CAD build for the part. Positions are in the model's coordinates, mm. A direction names the side the tool comes from. Give positions to 0.01 mm unless a question says otherwise; leave off trailing zeros. Order: outer loops, then holes, each group sorted by start corner. A loop starts at its lowest first (then second) coordinate and runs counter-clockwise, first axis right, second up. Notation, with made-up numbers: M -29,2.25 L 25,2.25 A21 ccw 25,21.25 Z; hole C 63,22.5 d11. An arc over 180 degrees is marked long. Put each result on its own line as item: value. Start each with the question number.
1) Cut at A-A (z = 12). Write the cut outline in (x, y).
2) Two-plate mould, pull along Y, no slides. Class faces 1 (the face through (2, 176, 2)), 2 (the face through (-2, 240, 7)), 3 (the face through (-2, 212, 0)): released by +Y, released by -Y, zero draft, split by the parting line, or undercut.
3) Drill centre lines: line 1 (X direction, y = 175.5, z = 10.25); line 2 (Y direction, x = 36.5, z = 11); line 3 (Z direction, x = 1.5, y = 170). Where is each one in solid material? Low to high. Write a range as [from, to].
4) Pin check, flat tip, straight feed: pin 1 (6.5 mm diameter, centred on x = 36.5, y = -175.5, fed in from -Z). Stop position of the tip, or through.
5) Tool access for faces 4 (the face through (2, -175, 2)), 5 (the face through (-2, 3, 15)): list every direction of +Z, -Z, +X, -X, +Y, -Y with a clear straight run to the whole face (end or side of a thin tool).
```python
from build123d import *

# Parameters (mm, degrees)
SKETCH_1_W          = 307
SKETCH_1_H          = 480
EXTRUDE_1_DEPTH     = 15
SKETCH_2_W          = 307
SKETCH_2_H          = 15
CUT_EXTRUDE_1_DEPTH = 2
CUT_EXTRUDE_2_DEPTH = 286.284507115
HOLE_WIZARD_M6_1_D  = 5


with BuildPart() as part:
    # 草图1 → 凸台-拉伸1 (new body)
    with BuildSketch(Plane.XY):
        Rectangle(SKETCH_1_W, SKETCH_1_H)
    extrude(amount=EXTRUDE_1_DEPTH)

    # 草图2 → 切除-拉伸1 (cut)
    with BuildSketch(Plane(origin=(0, 0, 0), x_dir=(-1, 0, 0), z_dir=(0, 0, -1))):
        with Locations((0, 175.5)):
            Rectangle(SKETCH_2_W, SKETCH_2_H)
        with Locations((0, -175.5)):
            Rectangle(SKETCH_2_W, SKETCH_2_H)
    extrude(amount=-CUT_EXTRUDE_1_DEPTH, mode=Mode.SUBTRACT)

    # 草图3 → 切除-拉伸2 (cut, through all)
    with BuildSketch(Plane(origin=(0, 0, 0), x_dir=(-1, 0, 0), z_dir=(0, 0, -1))):
        with BuildLine():
            ThreePointArc((153.5, -76.852130745), (256.256578441, -87.624910842), (311, 0))
            ThreePointArc((311, 0), (256.256578441, 87.624910842), (153.5, 76.852130745))
            Line((153.5, 76.852130745), (153.5, -76.852130745))
        make_face()
        with BuildLine():
            Line((153.5, -76.852130745), (153.5, 76.852130745))
            ThreePointArc((153.5, 76.852130745), (116, 0), (153.5, -76.852130745))
        make_face()
    extrude(amount=-CUT_EXTRUDE_2_DEPTH, mode=Mode.SUBTRACT)

    # M6 螺纹孔1 (through all)
    with Locations(Plane(origin=(0, 0, 2), x_dir=(-1, 0, 0), z_dir=(0, 0, -1))):
        with Locations((63.5, -175.5), (-36.5, -175.5), (-136.5, -175.5), (-136.5, 175.5), (-36.5, 175.5), (63.5, 175.5)):
            Hole(HOLE_WIZARD_M6_1_D / 2)


solid = part.part
```
Solution:
1. outline: M -153.5,-240 L 153.5,-240 L 153.5,240 L -153.5,240 L -153.5,76.85 A97.5 cw -153.5,-76.85 Z; hole C -63.5,-175.5 d5; hole C -63.5,175.5 d5; hole C 36.5,-175.5 d5; hole C 36.5,175.5 d5; hole C 136.5,-175.5 d5; hole C 136.5,175.5 d5
2. face 1: undercut
2. face 2: released by +Y
2. face 3: zero draft
3. line 1: [-153.5, -66], [-61, 34], [39, 134], [139, 153.5]
3. line 2: [-240, -178], [-173, 173], [178, 240]
3. line 3: [2, 15]
4. pin 1: z = 2
5. face 4: -Z, +X, -X
5. face 5: +Z, +X, -X, +Y, -Y
